Verification items for the finished model (mm, model axes). Face numbers are marked on the shaded views. A direction names the side the tool comes from. Round coordinates to 2 decimals unless told otherwise and drop trailing zeros. Order: outer loops, then holes, each group sorted by start corner. A loop starts at its lowest first (then second) coordinate and runs counter-clockwise, first axis right, second up. Notation, with made-up numbers: M 18.5,-0.75 L 52.5,-0.75 A28 cw 52.5,25.25 Z; hole C 66,50 d2. An arc over 180 degrees is marked long. Use CSV: the item, a comma, the result in double quotes. Start each with the question number.
Q1. Sectioned sample at A-A (x = 44.45). Enter the section's corners in (y, z), and give its area (3 significant figures).
Q2. Set-up check for the marked faces 4 and 5: record each of +Z, -Z, +X, -X, +Y, -Y from which the full face is reachable in a straight line by a thin tool's end or side.
Q3. Gauge pin test, flat ends, axial feed: pin 1 Ø4 at (x, z) = (17.5, 1.5) entering from +Y; pin 2 Ø4 at (y, z) = (24, 10.5) entering from +X; pin 3 Ø6 at (x, z) = (37, 4) entering from +Y. Record the tip position at first contact, or that the pin passes through.
Q4. Mould release check, pull along Y, two halves, no side actions. Record for the marked faces 1, 2 and 3: +Y half, -Y half, draft (parallel to the pull), parting line (faces both ways), or undercut.
Q5. Scan lines: line 1 (Y direction, x = 44.5, z = 6.5); line 2 (Y direction, x = 30.5, z = 9); line 3 (Y direction, x = 12.7, z = 4). Record each from-to range of solid material in increasing order.
Q6. Sectioned sample at B-B (z = 9.5). Enter the section's corners in (x, y).
```python
from build123d import *

# Parameters (mm, degrees)
SKETCH1_R           = 2.286
BOSS_EXTRUDE1_DEPTH = 12.7
FILLET2_R           = 3.81
FILLET3_R           = 2.54
SKETCH6_R           = 2.286
CUT_EXTRUDE4_DEPTH  = 68.870777217
FILLET4_R           = 0.508


with BuildPart() as part:
    # Sketch1 → Boss-Extrude1 (new body)
    with BuildSketch(Plane.XY):
        Polygon((7.613799027, 43.18), (0, 0), (50.8, 0), (50.8, 12.7), (25.4, 12.7), (15.233799027, 43.18), align=None)
        with Locations((11.876425153, 38.1)):
            Circle(SKETCH1_R, mode=Mode.SUBTRACT)
    extrude(amount=BOSS_EXTRUDE1_DEPTH)

    # Fillet2
    fillet2_edges = [part.edges().sort_by_distance(p)[0] for p in [
        (0, 0, 6.35),
        (7.613799027, 43.18, 6.35),
        (15.233799027, 43.18, 6.35),
        (25.4, 12.7, 6.35),
    ]]
    fillet(fillet2_edges, radius=FILLET2_R)

    # Fillet3
    fillet3_edges = [part.edges().sort_by_distance(p)[0] for p in [
        (50.8, 12.7, 6.35),
        (50.8, 0, 6.35),
    ]]
    fillet(fillet3_edges, radius=FILLET3_R)

    # Sketch6 → Cut-Extrude4 (cut, through all)
    with BuildSketch(Plane(origin=(0, 0, 0), x_dir=(-1, 0, 0), z_dir=(0, 0, -1))):
        with Locations((-44.45, 6.35)):
            Circle(SKETCH6_R)
        with Locations((-12.7, 6.35)):
            Circle(SKETCH6_R)
    extrude(amount=-CUT_EXTRUDE4_DEPTH, mode=Mode.SUBTRACT)

    # Fillet4
    fillet4_edges = [part.edges().sort_by_distance(p)[0] for p in [
        (11.64950248, 43.18, 0),
        (11.64950248, 43.18, 12.7),
        (26.400290594, 0, 0),
        (3.923557366, 22.251599557, 0),
        (20.316899513, 27.94, 0),
        (8.361747829, 42.288629328, 0),
        (1.62195186, 1.360979207, 0),
        (14.715699565, 42.46103665, 0),
        (20.316899513, 27.94, 12.7),
        (26.400290594, 0, 12.7),
        (3.923557366, 22.251599557, 12.7),
        (8.361747829, 42.288629328, 12.7),
        (1.62195186, 1.360979207, 12.7),
        (14.715699565, 42.46103665, 12.7),
        (25.918099462, 13.41896335, 0),
        (25.918099462, 13.41896335, 12.7),
        (50.8, 6.35, 0),
        (50.8, 6.35, 12.7),
        (38.202781345, 12.7, 0),
        (50.056051224, 11.956051224, 0),
        (50.056051224, 0.743948776, 0),
        (38.202781345, 12.7, 12.7),
        (50.056051224, 11.956051224, 12.7),
        (50.056051224, 0.743948776, 12.7),
    ]]
    fillet(fillet4_edges, radius=FILLET4_R)


solid = part.part
```
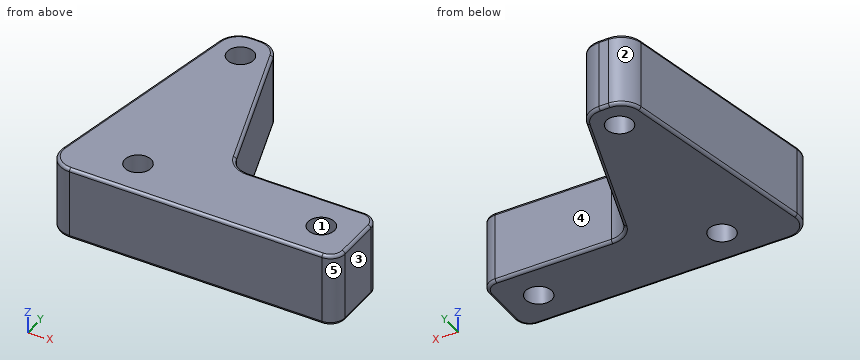
Verdict:
1,outline,"M 0,0.51 A0.51 ccw 0.51,0 L 4.06,0 L 4.06,12.7 L 0.51,12.7 A0.51 ccw 0,12.19 Z; M 8.64,0 L 12.19,0 A0.51 ccw 12.7,0.51 L 12.7,12.19 A0.51 ccw 12.19,12.7 L 8.64,12.7 Z"
1,area,"103 mm²"
2,face 4,"+Z, -Z, +X, +Y"
2,face 5,"+Z, -Z, +X, -Y"
3,pin 1,"stops at y = 41.7"
3,pin 2,"stops at x = 22.3"
3,pin 3,"stops at y = 12.7"
4,face 1,"undercut"
4,face 2,"+Y half"
4,face 3,"draft"
5,line 1,"y = 0 to 4.06, 8.64 to 12.7"
5,line 2,"y = 0 to 12.7"
5,line 3,"y = 0 to 4.06, 8.64 to 35.97, 40.23 to 43.17"
6,outline,"M 0.79,4.47 A3.81 ccw 4.54,0 L 48.26,0 A2.54 ccw 50.8,2.54 L 50.8,10.16 A2.54 ccw 48.26,12.7 L 28.15,12.7 A3.81 cw 24.53,15.3 L 16.1,40.58 A3.81 ccw 12.49,43.18 L 10.81,43.18 A3.81 ccw 7.06,40.03 Z; hole C 11.88,38.1 d4.57; hole C 12.7,6.35 d4.57; hole C 44.45,6.35 d4.57"
